```python
from build123d import *

# Parameters (mm, degrees)
SKETCH3_R          = 1.905
CUT_EXTRUDE1_DEPTH = 21.329919626


with BuildPart() as part:
    # Sketch2 → Loft1 section 0
    with BuildSketch(Plane(origin=(0, 12.7, 0), x_dir=(1, 0, 0), z_dir=(0, 1, 0))):
        with BuildLine():
            Line((-6.35, -6.35), (6.35, -6.35))
            Line((6.35, -6.35), (6.35, 6.35))
            Line((6.35, 6.35), (-6.35, 6.35))
            Line((-6.35, 6.35), (-6.35, -6.35))
        make_face()
    # Sketch1 → Loft1 section 1
    with BuildSketch(Plane(origin=(0, 0, 0), x_dir=(1, 0, 0), z_dir=(0, 1, 0))):
        with BuildLine():
            Line((-12.7, -9.525), (12.7, -9.525))
            Line((12.7, -9.525), (12.7, 9.525))
            Line((12.7, 9.525), (-12.7, 9.525))
            Line((-12.7, 9.525), (-12.7, -9.525))
        make_face()
    loft()

    # Sketch3 → Cut-Extrude1 (cut, through all)
    with BuildSketch(Plane(origin=(0, 12.7, 0), x_dir=(1, 0, 0), z_dir=(0, 1, 0))):
        with Locations(Location((0, 0, 0), (0, 0, 270))):
            Circle(SKETCH3_R)
    extrude(amount=-CUT_EXTRUDE1_DEPTH, mode=Mode.SUBTRACT)


solid = part.part
```
Here's how the part is built. I have some questions about the finished solid (model axes, mm). Coordinates: 2 decimals unless noted, no trailing zeros. One line per question, with ' | ' between items. Start each with the question number.
1. Please list where these lines run through material, in increasing order: line 1 along X through (y, z) = (3.75, 0) (3 decimals); line 2 along X through (y, z) = (6.75, 0) (3 decimals); line 3 along Y through (x, z) = (11.75, 0.5). Write a range as [from, to].
2. I'm going to push flat-ended pins straight in: pin 1 Ø2 at (x, y) = (7.5, 8.5) entering from +Z; pin 2 Ø1.5 at (y, z) = (2, 2) entering from -X (3 decimals); pin 3 Ø2 at (y, z) = (10, 4.5) entering from +X. Where does each tip first touch, or does it pass through?
3. If we mould it in two halves opening along Z, with no side actions, what happens to faces 1 (the cylindrical face through (1.89, 6.44, -0.25)), 2 (the flat face through (-1, 12.7, 2))? For each: released by +Z, released by -Z, zero draft, split by the parting line, or undercut.
Model answer:
1) line 1: x = [-10.825, -1.905], [1.905, 10.825] | line 2: x = [-9.325, -1.905], [1.905, 9.325] | line 3: y = [0, 1.9]
2) pin 1: stops at z = 7.65 | pin 2: stops at x = -12.075 | pin 3: stops at x = 8.2
3) face 1: undercut | face 2: zero draft
